Part model, mm, in its own coordinate system. A direction names the side the tool comes from. Round coordinates to 2 decimals unless told otherwise and drop trailing zeros. Write each loop counter-clockwise with the first axis right and the second up, starting at its lowest first coordinate (ties: lowest second). Pieces come first, ordered by that corner, then holes. Notation, with made-up numbers: (8.25, 44) -> (46.25, 44) arc R31 cw to (46.25, 68) -> close; hole circle Ø2 at (-11, 78). An arc over 180 degrees is marked (long way). Return JSON: item names as keys, results as strings. Group by question number.
Autodesk Inventor part; units mm, degrees
ref_plane "Work Plane2" through (0, 34, 0) normal (0, -1, 0) x (1, 0, 0)
ref_plane "YZ Plane" through (0, 0, 0) normal (1, 0, 0) x (0, 1, 0)
ref_plane "XZ Plane" through (0, 0, 0) normal (0, 1, 0) x (-1, 0, 0)
sketch "Sketch1" plane through (0, 0, 0) normal (0, 1, 0) x (-1, 0, 0)
  circle A0 centre (0, 0) radius 18
  arc A1 (19, 0) -> (0, -19) centre (0, 0) ccw
  line L0 (19, -19) -> (0, -19) construction
  line L1 (-19, -19) -> (-19, 19)
  line L2 (-19, 19) -> (0, 19)
  line L3 (19, 19) -> (19, 0) construction
  line L4 (19, -19) -> (-19, 19) construction
  line L5 (-19, -19) -> (19, 19) construction
  line L6 (0, -19) -> (-19, -19)
  line L7 (19, 0) -> (19, -19) construction
  arc A2 (13.435, -13.435) -> (19, 0) centre (0, 0) ccw
  arc A3 (0, -19) -> (13.435, -13.435) centre (0, 0) ccw
  line L8 (0, 19) -> (19, 19) construction
  dimension "d0" = 36
  dimension "d1" = 38
extrude "Extrusion1" add sketch "Sketch1" along normal blind 68
ref_plane "Work Plane2" through (0, 34, 0) normal (0, -1, 0) x (1, 0, 0)
sketch "Sketch10" plane through (0, 68, 0) normal (0, 1, 0) x (1, 0, 0)
  line L0 (19, -19) -> (19, 19)
  line L1 (19, 19) -> (12.7279, 12.7279) construction
  circle A0 centre (0, 0) radius 18
  line L2 (0, -19) -> (19, -19)
  line L3 (19, -19) -> (12.7279, -12.7279) construction
  circle A1 centre (15.864, 15.864) radius 1.55
  circle A2 centre (15.864, -15.864) radius 1.55
  dimension "d21" = 3.1
  dimension "d22" = 3.1
extrude "Extrusion5" cut sketch "Sketch10" against normal through all contours A1 | A2
sketch "Sketch11" plane through (19, 0, 19) normal (1, 0, 0) x (0, 0, -1)
  line L0 (0, 68) -> (38, 68)
  line L1 (0, 0) -> (38, 0)
  line L2 (0, 68) -> (38, 0) construction
  line L3 (38, 68) -> (0, 0) construction
  line L4 (36.414, 68) -> (36.414, 0)
  line L5 (1.586, 51.5) -> (36.414, 51.5)
  line L6 (36.414, 51.5) -> (36.414, 16.5)
  line L7 (36.414, 16.5) -> (1.586, 16.5)
  line L8 (1.586, 16.5) -> (1.586, 51.5)
  line L9 (1.586, 51.5) -> (36.414, 16.5) construction
  line L10 (36.414, 51.5) -> (1.586, 16.5) construction
  point P0 (19, 0)
  point P1 (19, 34)
  dimension "d25" = 35
extrude "Extrusion6" cut sketch "Sketch11" against normal up to next
sketch "Sketch12" plane through (19, 0, 19) normal (1, 0, 0) x (0, 0, -1)
  line L0 (38, 0) -> (38, 68)
  line L1 (36.414, 16.5) -> (36.414, 0)
  line L2 (38, 68) -> (36.414, 68)
  line L3 (36.414, 68) -> (36.414, 13.5)
  line L4 (36.414, 13.5) -> (38, 13.5)
  line L5 (38, 13.5) -> (38, 68)
  line L6 (1.586, 16.5) -> (1.586, 0)
  line L7 (0, 68) -> (1.586, 68)
  line L8 (1.586, 68) -> (1.586, 13.5)
  line L9 (1.586, 13.5) -> (0, 13.5)
  line L10 (0, 13.5) -> (0, 68)
  point P0 (38, 13.5)
  dimension "d33" = 54.5
extrude "Extrusion7" add sketch "Sketch12" along normal blind 2.5
sketch "Sketch13" plane through (19, 16.5, 17.414) normal (0, 1, 0) x (1, 0, 0)
  line L0 (0, 34.8279) -> (0, 0)
  line L1 (0, 34.8279) -> (-3.136, 34.8279)
  line L2 (-3.136, 34.8279) -> (-14.4443, 34.8279)
  arc A0 (-14.4443, 0) -> (-14.4443, 34.8279) centre (-19, 17.414) ccw
  circle A1 centre (-3.136, 33.2779) radius 1.55
  circle A2 centre (-3.136, 33.2779) radius 1.55
  circle A3 centre (-3.136, 33.2779) radius 2.5 construction
  line L3 (0, 30.7779) -> (-6.9416, 30.7779)
  circle A4 centre (-19, 17.414) radius 18
  line L4 (0, 34.8279) -> (-14.4443, 34.8279)
  line L5 (0, 34.8279) -> (0, 30.7779)
  line L6 (-19, 17.414) -> (-15.9745, 17.414) construction
  line L7 (0, 0) -> (-3.136, 0)
  line L8 (-3.136, 0) -> (-14.4443, 0)
  circle A5 centre (-3.136, 1.55) radius 1.55
  circle A6 centre (-3.136, 1.55) radius 1.55
  circle A7 centre (-3.136, 1.55) radius 2.5 construction
  line L9 (0, 4.05) -> (-6.9416, 4.05)
  line L10 (0, 0) -> (-14.4443, 0)
  line L11 (0, 0) -> (0, 4.05)
  point P0 (0, 4.05)
  point P1 (-6.9416, 4.05)
  dimension "d30" = 5
extrude "Extrusion8" add sketch "Sketch13" along normal up to next contours L0 L3 A0 L2 L1 | L0 L7 L8 A0 L9
properties part number "Tubo" material "ABS Plastic"
Item 1: Cut at D-D (y = 45). State how many separate pieces and enclosed holes the cut face has, then the cut area to 3 significant figures.
Item 2: Flat gauge pins, fed straight in: P1, Ø1.7, axis at x = 20, z = 18.5, coming from the -Y side; P2, Ø1.9, axis at x = 15.864, z = -15.864, coming from the +Y side; P3, Ø2, axis at y = 24, z = 13.5, coming from the -X side; P4, Ø2, axis at x = -8.5, y = 32.5, coming from the +Z side. Where does each tip first touch, or does it go through?
Item 3: Wall check: L1, parallel to Z at x = 0, y = 31; L2, parallel to Z at x = 17.5, y = 46; L3, parallel to Z at x = 14.5, y = 39. Give the ranges that are in metal, low to high.
Item 4: Cut at A-A (x = -7.5). Write the cut outline in (y, z), then the cut area to 3 significant figures.
Item 5: Cut at B-B (z = 12.5). Write the cut outline in (x, y), then the cut area to 3 significant figures.
Item 6: Which spindle directions (+Z, -Z, +X, -X, +Y, -Y) get a long thin tool onto all of the face, cutting with end or side? Do faces 4 (the face through (20, 41, -17.414)), 5 (the face through (18.7, 51.5, 0.2)), 6 (the face through (20, 13.5, 18)). Say none if no direction does.
Item 7: Cut at C-C (y = 61). Write the cut outline in (x, z) (3 decimals), then the cut area to 3 significant figures.
Item 8: Two-plate mould, pull along X, no slides. Class faces 1 (the face through (8.497, 33.755, -15.868)), 2 (the face through (16, 34, 13.364)), 3 (the face through (-17.593, 33.524, -7.174)): released by +X, released by -X, zero draft, split by the parting line, or undercut.
Checks:
{
 "1": {"separate pieces": "1", "enclosed holes": "2", "area": "188 mm2"},
 "2": {"P1": "stops at y = 13.5", "P2": "passes through", "P3": "stops at x = -14.31", "P4": "stops at z = 17.46"},
 "3": {"L1": "z = -19 to -18, 18 to 19", "L2": "z = -19 to -13.36, 13.36 to 19", "L3": "z = -19 to -16.6, -15.13 to -13.36, 13.36 to 15.13, 16.6 to 19"},
 "4": {"outline": "(0, -17.46) -> (68, -17.46) -> (68, -16.36) -> (0, -16.36) -> close; (0, 16.36) -> (68, 16.36) -> (68, 17.46) -> (0, 17.46) -> close", "area": "149 mm2"},
 "5": {"outline": "(-14.31, 0) -> (-12.95, 0) -> (-12.95, 68) -> (-14.31, 68) -> close; (12.95, 0) -> (19, 0) -> (19, 16.5) -> (12.95, 16.5) -> close; (12.95, 51.5) -> (19, 51.5) -> (19, 68) -> (12.95, 68) -> close", "area": "292 mm2"},
 "6": {"face 4": "+X, +Y, -Y", "face 5": "+X", "face 6": "+Z, -Z, +X, -Y"},
 "7": {"outline": "(-19, 0) arc R19 ccw to (-13.435, -13.435) arc R19 ccw to (0, -19) -> (21.5, -19) -> (21.5, -17.414) -> (19, -17.414) -> (19, 17.414) -> (21.5, 17.414) -> (21.5, 19) -> (0, 19) arc R19 ccw to start; hole circle Ø36 at (0, 0); hole circle Ø3.1 at (15.864, -15.864); hole circle Ø3.1 at (15.864, 15.864)", "area": "264 mm2"},
 "8": {"face 1": "undercut", "face 2": "zero draft", "face 3": "released by -X"}
}
